Here's how the part is built. I have some questions about the finished solid (model axes, mm). Face numbers are marked on the shaded views. A direction names the side the tool comes from. Coordinates: 2 decimals unless noted, no trailing zeros. Write each loop counter-clockwise with the first axis right and the second up, starting at its lowest first coordinate (ties: lowest second). Pieces come first, ordered by that corner, then holes.
Item 1: I'm going to push flat-ended pins straight in: P1, Ø10, axis at x = 20, z = 9.5, coming from the -Y side; P2, Ø4, axis at x = -33.5, z = -6, coming from the -Y side; P3, Ø7.5, axis at x = -33.5, y = -7.5, coming from the +Z side. Where does each tip first touch, or does it pass through?
Item 2: I want a section at B-B (z = 1). Please give me the cut outline in (x, y).
Item 3: I want a section at C-C (y = -55). Please give me the cut outline in (x, z) (3 decimals).
Item 4: I want a section at A-A (y = -23.5). Please give me the cut outline in (x, z), and give its area (3 significant figures).
Item 5: Please list where these lines run through material, in increasing order: line 1 (X direction, y = -25, z = -2); line 2 (Y direction, x = -6, z = 4); line 3 (Y direction, x = 40.1, z = 0).
Item 6: I want a section at D-D (z = -10.5). Please give me the cut outline in (x, y).
Item 7: For the marked faces 4, 5 and 6, which set-ups out of +Z, -Z, +X, -X, +Y, -Y let a thin tool reach every point of the face, with its end or its side?
Item 8: If we mould it in two halves opening along X, with no side actions, what happens to the marked faces 1, 2 and 3? For each: pulls with the +X half, pulls with the -X half, needs draft (parallel to the pull), parting line crosses it, or undercut.
from build123d import *

# Parameters (mm, degrees)
BRACKET_U_SHAPE_DEPTH              = 12.5
SKETCH3_R                          = 17.25
MOTOR_RING_DEPTH                   = 5
MOTOR_RING_FILLETS_15MM_R          = 15
U_BRACKET_BOTTOM_ROUNDING_12_5MM_R = 12.5
SKETCH4_R                          = 17.25
TILT_MOTOR_TAB_DEPTH               = 5
TILT_MOTOR_TAB_FILLETS_15MM_R      = 15
SKETCH6_R                          = 8
BEARING_HOLE_CUT_DEPTH             = 106.925091456


with BuildPart() as part:
    # Sketch2 → Bracket U-shape (new, symmetric)
    with BuildSketch(Plane.XY):
        with BuildLine():
            Line((-37.5, -67.25), (-37.5, -10))
            ThreePointArc((-37.5, -10), (-34.571067812, -2.928932188), (-27.5, 0))
            Line((-27.5, 0), (27.5, 0))
            ThreePointArc((27.5, 0), (34.571067812, -2.928932188), (37.5, -10))
            Line((37.5, -10), (37.5, -67.25))
            Line((37.5, -67.25), (42.5, -67.25))
            Line((42.5, -67.25), (42.5, -10))
            ThreePointArc((42.5, -10), (38.106601718, 0.606601718), (27.5, 5))
            Line((27.5, 5), (-27.5, 5))
            ThreePointArc((-27.5, 5), (-38.106601718, 0.606601718), (-42.5, -10))
            Line((-42.5, -10), (-42.5, -67.25))
            Line((-42.5, -67.25), (-37.5, -67.25))
        make_face()
    extrude(amount=BRACKET_U_SHAPE_DEPTH, both=True)

    # Sketch3 → Motor ring (add)
    with BuildSketch(Plane(origin=(0, 5, 0), x_dir=(1, 0, 0), z_dir=(0, 1, 0))):
        Circle(SKETCH3_R)
    extrude(amount=-MOTOR_RING_DEPTH)

    # Motor ring fillets 15mm
    motor_ring_fillets_15mm_edges = [part.edges().sort_by_distance(p)[0] for p in [
        (11.887493428, 2.5, -12.5),
        (-11.887493428, 2.5, -12.5),
        (-11.887493428, 2.5, 12.5),
        (11.887493428, 2.5, 12.5),
    ]]
    fillet(motor_ring_fillets_15mm_edges, radius=MOTOR_RING_FILLETS_15MM_R)

    # U bracket bottom rounding 12.5mm
    u_bracket_bottom_rounding_12_5mm_edges = [part.edges().sort_by_distance(p)[0] for p in [
        (40, -67.25, 12.5),
        (40, -67.25, -12.5),
        (-40, -67.25, -12.5),
        (-40, -67.25, 12.5),
    ]]
    fillet(u_bracket_bottom_rounding_12_5mm_edges, radius=U_BRACKET_BOTTOM_ROUNDING_12_5MM_R - 0.0001)  # a hair under: the kernel refuses the full size

    # Sketch4 → Tilt motor tab (add)
    with BuildSketch(Plane.ZY.offset(42.5)):
        with Locations((0, -50)):
            Circle(SKETCH4_R)
    extrude(amount=-TILT_MOTOR_TAB_DEPTH)

    # Tilt motor tab fillets 15mm
    tilt_motor_tab_fillets_15mm_edges = [part.edges().sort_by_distance(p)[0] for p in [
        (-40, -38.112506572, 12.5),
        (-40, -38.112506572, -12.5),
    ]]
    fillet(tilt_motor_tab_fillets_15mm_edges, radius=TILT_MOTOR_TAB_FILLETS_15MM_R)

    # Sketch6 → Bearing hole cut (cut, through all)
    with BuildSketch(Plane.ZY.offset(-37.5)):
        with Locations((0, -50)):
            Circle(SKETCH6_R)
        with BuildLine():
            Line((12.5, -54.75), (12.5, -50))
            ThreePointArc((12.5, -50), (0, -62.5), (-12.5, -50))
            Line((-12.5, -50), (-12.5, -54.75))
            ThreePointArc((-12.5, -54.75), (-8.838834765, -63.588834765), (0, -67.25))
            ThreePointArc((0, -67.25), (8.838834765, -63.588834765), (12.5, -54.75))
        make_face()
    extrude(amount=-BEARING_HOLE_CUT_DEPTH, mode=Mode.SUBTRACT)


with BuildPart() as bearing_hole_cut_kept_piece:
    # of the separate pieces the step leaves, the one the design keeps (bearing_hole_cut_pieces_kept)
    add(part.part.solids().sort_by_distance((-37.5, -33.153264411, -12.5))[0])


solid = bearing_hole_cut_kept_piece.part
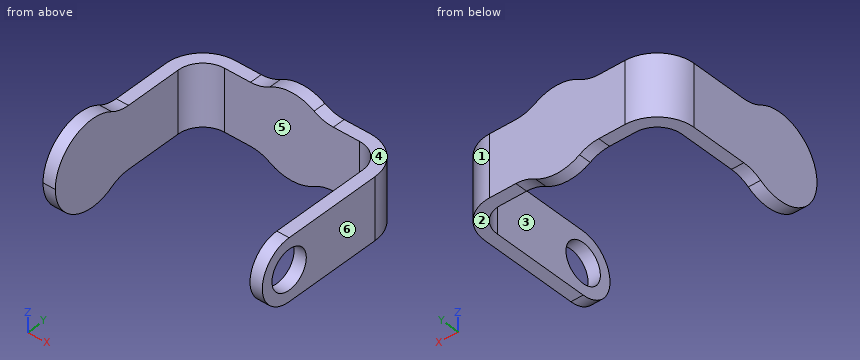
Answer:
1. P1: stops at y = 0
1. P2: stops at y = -4
1. P3: stops at z = 12.5
2. outline: (-42.5, -67.22) - (-37.5, -67.22) - (-37.5, -10) arc R10 cw to (-27.5, 0) - (27.5, 0) arc R10 cw to (37.5, -10) - (37.5, -42.06) - (42.5, -42.06) - (42.5, -10) arc R15 ccw to (27.5, 5) - (-27.5, 5) arc R15 ccw to (-42.5, -10) - close; (37.5, -62.46) - (42.5, -62.46) - (42.5, -57.94) - (37.5, -57.94) - close
3. outline: (-42.5, -16.509) - (-37.5, -16.509) - (-37.5, 16.509) - (-42.5, 16.509) - close; (37.5, -11.456) - (42.5, -11.456) - (42.5, -6.245) - (37.5, -6.245) - close; (37.5, 6.245) - (42.5, 6.245) - (42.5, 11.456) - (37.5, 11.456) - close
4. outline: (-42.5, -12.5) - (-37.5, -12.5) - (-37.5, 12.5) - (-42.5, 12.5) - close; (37.5, -12.5) - (42.5, -12.5) - (42.5, 12.5) - (37.5, 12.5) - close
4. area: 250 mm2
5. line 1: x = -42.5 to -37.5, 37.5 to 42.5
5. line 2: y = 0 to 5
5. line 3: y = -62.5 to -58, -42 to -1.86
6. outline: (-42.5, -63.69) - (-37.5, -63.69) - (-37.5, -10) arc R10 cw to (-27.5, 0) - (27.5, 0) arc R10 cw to (37.5, -10) - (37.5, -56.78) - (42.5, -56.78) - (42.5, -10) arc R15 ccw to (27.5, 5) - (-27.5, 5) arc R15 ccw to (-42.5, -10) - close
7. face 4: +Z, +X, +Y, -Y
7. face 5: +Z, -Z, -Y
7. face 6: +Z, -Z, +X, +Y, -Y
8. face 1: pulls with the +X half
8. face 2: needs draft
8. face 3: undercut
